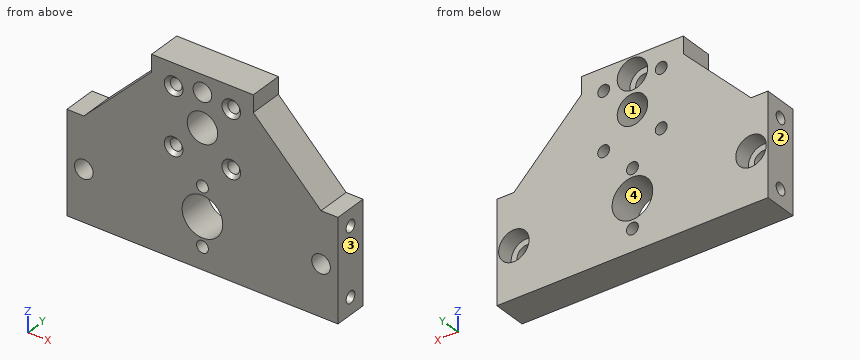
```python
from build123d import *

# Parameters (mm, degrees)
SKETCH1_W           = 80
SKETCH1_H           = 30
SKETCH1_R           = 1.75
SKETCH1_R_2         = 6
SKETCH1_R_3         = 2.75
BOSS_EXTRUDE1_DEPTH = 10
SKETCH4_W           = 25
SKETCH4_H           = 10
BOSS_EXTRUDE3_DEPTH = 15
SKETCH5_R           = 2.75
CUT_EXTRUDE1_DEPTH  = 30
CHAMFER2_SIZE       = 20
SKETCH6_R           = 1.75
SKETCH6_R_2         = 4.5
CUT_EXTRUDE2_DEPTH  = 30
SKETCH8_R           = 1.75
CUT_EXTRUDE3_DEPTH  = 91
CUT_EXTRUDE13_START = -5
SKETCH12_R          = 4.5
CUT_EXTRUDE13_DEPTH = 53.445626552
CHAMFER3_SIZE       = 1


with BuildPart() as part:
    # Sketch1 → Boss-Extrude1 (new body)
    with BuildSketch(Plane(origin=(0, 0, 0), x_dir=(1, 0, 0), z_dir=(0, 1, 0))):
        Rectangle(SKETCH1_W, SKETCH1_H)
        with Locations(Location((0, 8.5, 0), (0, 0, 270))):
            Circle(SKETCH1_R, mode=Mode.SUBTRACT)
        with Locations(Location((0, -8.5, 0), (0, 0, 270))):
            Circle(SKETCH1_R, mode=Mode.SUBTRACT)
        with Locations(Location((0, 0, 0), (0, 0, 270))):
            Circle(SKETCH1_R_2, mode=Mode.SUBTRACT)
        with Locations(Location((-35, 0, 0), (0, 0, 270))):
            Circle(SKETCH1_R_3, mode=Mode.SUBTRACT)
        with Locations(Location((35, 0, 0), (0, 0, 270))):
            Circle(SKETCH1_R_3, mode=Mode.SUBTRACT)
    extrude(amount=BOSS_EXTRUDE1_DEPTH)

    # Sketch4 → Boss-Extrude3 (add, symmetric)
    with BuildSketch(Plane(origin=(0, 0, 0), x_dir=(0, 0, -1), z_dir=(1, 0, 0))):
        with Locations((-27.5, 5)):
            Rectangle(SKETCH4_W, SKETCH4_H)
    extrude(amount=BOSS_EXTRUDE3_DEPTH, both=True)

    # Sketch5 → Cut-Extrude1 (cut)
    with BuildSketch(Plane(origin=(0, 10, 0), x_dir=(1, 0, 0), z_dir=(0, 1, 0))):
        with Locations(Location((0, -35, 0), (0, 0, 270))):
            Circle(SKETCH5_R)
    extrude(amount=-CUT_EXTRUDE1_DEPTH, mode=Mode.SUBTRACT)

    # Chamfer2
    chamfer2_edges = [part.edges().sort_by_distance(p)[0] for p in [
        (-15, 5, 15),
        (15, 5, 15),
    ]]
    chamfer(chamfer2_edges, length=CHAMFER2_SIZE)

    # Sketch6 → Cut-Extrude2 (cut)
    with BuildSketch(Plane(origin=(0, 10, 0), x_dir=(1, 0, 0), z_dir=(0, 1, 0))):
        with Locations(Location((-8.5, -16.5, 0), (0, 0, 270))):
            Circle(SKETCH6_R)
        with Locations(Location((8.5, -16.5, 0), (0, 0, 270))):
            Circle(SKETCH6_R)
        with Locations(Location((8.5, -33.5, 0), (0, 0, 270))):
            Circle(SKETCH6_R)
        with Locations(Location((-8.5, -33.5, 0), (0, 0, 270))):
            Circle(SKETCH6_R)
        with Locations(Location((0, -25, 0), (0, 0, 270))):
            Circle(SKETCH6_R_2)
    extrude(amount=-CUT_EXTRUDE2_DEPTH, mode=Mode.SUBTRACT)

    # Sketch8 → Cut-Extrude3 (cut, through all)
    with BuildSketch(Plane(origin=(40, 0, 0), x_dir=(0, 0, -1), z_dir=(1, 0, 0))):
        with Locations((-10, 5)):
            Circle(SKETCH8_R)
        with Locations((10, 5)):
            Circle(SKETCH8_R)
    extrude(amount=-CUT_EXTRUDE3_DEPTH, mode=Mode.SUBTRACT)

    # Sketch12 → Cut-Extrude13 (cut, through all)
    with BuildSketch(Plane.XZ.offset(CUT_EXTRUDE13_START)):
        with Locations(Location((0, 35, 0), (0, 0, 270))):
            Circle(SKETCH12_R)
        with Locations(Location((35, 0, 0), (0, 0, 270))):
            Circle(SKETCH12_R)
        with Locations(Location((-35, 0, 0), (0, 0, 270))):
            Circle(SKETCH12_R)
    extrude(amount=-CUT_EXTRUDE13_DEPTH, mode=Mode.SUBTRACT)

    # Chamfer3
    chamfer3_edges = [part.edges().sort_by_distance(p)[0] for p in [
        (-8.5, 0, 14.75),
        (8.5, 0, 31.75),
        (-8.5, 0, 31.75),
        (8.5, 0, 14.75),
    ]]
    chamfer(chamfer3_edges, length=CHAMFER3_SIZE)


solid = part.part
```
Geometry: final body of the model. Coordinates: model frame, mm. Face numbers are marked on the shaded views. Coordinates: 2 decimals unless noted, no trailing zeros. Order: outer loops, then holes, each group sorted by start corner. A loop starts at its lowest first (then second) coordinate and runs counter-clockwise, first axis right, second up. Notation, with made-up numbers: M 52,3 L 58,3 A27 ccw 58,36 Z; hole C -27.5,41.5 d11. An arc over 180 degrees is marked long. Answer in a Markdown table with one row per item. Add a question column.
Q1. Section query D-D on z = 16.5. Return the cut outline in (x, y), and give its area (3 significant figures).
Q2. Line query: L1, parallel to X at y = 7.1, z = 0; L2, parallel to Y at x = 5, z = 10; L3, parallel to X at y = 1.95, z = 0. Output: solid intervals per line, ascending.
Q3. Section query C-C on x = -20. Return the cut outline in (y, z).
Q4. Contact query for flat-ended pins moving along their axis: P1, Ø4.5, axis at x = 0, z = 8.5, coming from the -Y side; P2, Ø5.5, axis at x = 38.5, y = 6.5, coming from the +Z side; P3, Ø3, axis at x = 8.5, z = 33.5, coming from the +Y side; P4, Ø1.5, axis at y = 3, z = 38.5, coming from the -X side. Output: stop coordinate, or through.
Q5. Section query A-A on z = 0. Return the cut outline in (x, y), and give its area (3 significant figures).
Q6. Section query B-B on y = 7.75. Count the separate pieces of the cut face and the enclosed holes in it, and give its area (3 significant figures).
Q7. Mould query, pull axis X, two halves, no side actions, for the marked faces 1, 2, 3 and 4. Classes: released by +X, released by -X, zero draft, split by the parting line, or undercut.
Completed:
| question | item | result |
|---|---|---|
| 1 | outline | M -33.5,0 L -11.25,0 L -10.25,1 L -10.25,10 L -33.5,10 Z; M -6.75,1 L -5.75,0 L 5.75,0 L 6.75,1 L 6.75,10 L -6.75,10 Z; M 10.25,1 L 11.25,0 L 33.5,0 L 33.5,10 L 10.25,10 Z |
| 1 | area | 598 mm2 |
| 2 | L1 | x = -40 to -39.5, -30.5 to -6, 6 to 30.5, 39.5 to 40 |
| 2 | L2 | y = 0 to 3.25, 6.75 to 10 |
| 2 | L3 | x = -40 to -37.75, -32.25 to -6, 6 to 32.25, 37.75 to 40 |
| 3 | outline | M 0,-15 L 10,-15 L 10,30 L 0,30 Z; hole C 5,-10 d3.5; hole C 5,10 d3.5 |
| 4 | P1 | stops at y = 0 |
| 4 | P2 | stops at z = 15 |
| 4 | P3 | passes through |
| 4 | P4 | stops at x = -15 |
| 5 | outline | M -40,0 L -37.75,0 L -37.75,5 L -39.5,5 L -39.5,10 L -40,10 Z; M -32.25,0 L -6,0 L -6,10 L -30.5,10 L -30.5,5 L -32.25,5 Z; M 6,0 L 32.25,0 L 32.25,5 L 30.5,5 L 30.5,10 L 6,10 Z; M 37.75,0 L 40,0 L 40,10 L 39.5,10 L 39.5,5 L 37.75,5 Z |
| 5 | area | 535 mm2 |
| 6 | separate pieces | 1 |
| 6 | enclosed holes | 11 |
| 6 | area | 3,120 mm2 |
| 7 | face 1 | undercut |
| 7 | face 2 | released by -X |
| 7 | face 3 | released by +X |
| 7 | face 4 | undercut |
